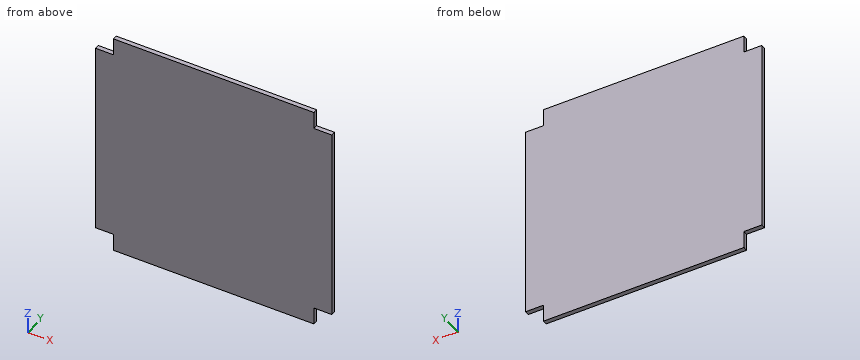
```python
from build123d import *

# Parameters (mm, degrees)
SKETCH1_W           = 530
SKETCH1_H           = 530
BOSS_EXTRUDE1_DEPTH = 10
SKETCH2_W           = 40
SKETCH2_H           = 40
CUT_EXTRUDE1_DEPTH  = 11


with BuildPart() as part:
    # Sketch1 → Boss-Extrude1 (new body)
    with BuildSketch(Plane(origin=(0, 0, 0), x_dir=(1, 0, 0), z_dir=(0, 1, 0))):
        Rectangle(SKETCH1_W, SKETCH1_H)
    extrude(amount=BOSS_EXTRUDE1_DEPTH)

    # Sketch2 → Cut-Extrude1 (cut, through all)
    with BuildSketch(Plane(origin=(0, 10, 0), x_dir=(1, 0, 0), z_dir=(0, 1, 0))):
        with Locations((-245, 245)):
            Rectangle(SKETCH2_W, SKETCH2_H)
        with Locations((245, 245)):
            Rectangle(SKETCH2_W, SKETCH2_H)
        with Locations((-245, -245)):
            Rectangle(SKETCH2_W, SKETCH2_H)
        with Locations((245, -245)):
            Rectangle(SKETCH2_W, SKETCH2_H)
    extrude(amount=-CUT_EXTRUDE1_DEPTH, mode=Mode.SUBTRACT)


solid = part.part
```
Source: CAD feature listing. Evaluate the final solid. Frame: model axes, mm. Coordinates: 2 decimals unless noted, no trailing zeros. Loops run counter-clockwise (first coordinate to the right, second up) from the corner with the lowest first, then second, coordinate; pieces in that order, holes last. Notation, with made-up numbers: M 57,11.5 L 77,11.5 A21 cw 77,43.5 Z; hole C -26.75,26.5 d11. An arc over 180 degrees is marked long. Put each result on its own line as item: value. Start each with the question number.
1) Ray query, L1, parallel to Z at x = -241, y = 2.5. Return the intervals inside material, ascending. Write a range as from..to.
2) Contact query for flat-ended pins moving along their axis: pin 1 Ø5 at (y, z) = (5.5, 241.5) entering from +X; pin 2 Ø3 at (x, y) = (-239.5, 3.5) entering from +Z; pin 3 Ø12 at (x, z) = (-184, 106.5) entering from -Y. Output: stop coordinate, or through.
3) Cut plane A-A on y = 6.75. Return the cut outline in (x, z), then the cut area to 4 significant figures.
The answers:
1. L1: z = -225..225
2. pin 1: stops at x = 225
2. pin 2: stops at z = 225
2. pin 3: stops at y = 0
3. outline: M -265,-225 L -225,-225 L -225,-265 L 225,-265 L 225,-225 L 265,-225 L 265,225 L 225,225 L 225,265 L -225,265 L -225,225 L -265,225 Z
3. area: 274,500 mm²
